Study the drawing (mm; zero at the part's minimum x, y, z) and answer. Round coordinates to 2 decimals unless told otherwise and drop trailing zeros. Order: outer loops, then holes, each group sorted by start corner. A loop starts at its lowest first (then second) coordinate and runs counter-clockwise, first axis right, second up. Notation, with made-up numbers: M 87,39 L 129,39 A21 ccw 129,47 Z; hole C 84.25,61.25 d7. An arc over 180 degrees is marked long. Put each result on its own line as item: value. Start each with the question number.
1. The part is cut by section C-C (y = 1.5). Give the vertices of the cut face in (x, z), then the cut area to 3 significant figures.
2. The mould has two halves that part along X. Classify the marked faces 1, 2 and 3: +X half, -X half, draft (parallel to the pull), parting line (faces both ways), or undercut.
3. Consider line 1 (Z direction, x = 21.5, y = 4); line 2 (X direction, y = 10.75, z = 27.5); line 3 (X direction, y = 4, z = 18). Determine where each line is inside the solid, lowest interval first.
4. The part is cut by section B-B (z = 13.5). Give the vertices of the cut face in (x, y), then the cut area to 3 significant figures.
5. Each of these flat-tipped pins is pushed along its axis until it touches: pin 1 Ø6 at (y, z) = (4, 35) entering from -X; pin 2 Ø2 at (x, y) = (37.5, 8.5) entering from +Z; pin 3 Ø2 at (y, z) = (11.5, 15.5) entering from -X; pin 4 Ø19 at (x, z) = (16, 23) entering from -Y. Where does it stop, or does it pass through?
6. The part is cut by section A-A (x = 15.5). Give the vertices of the cut face in (y, z).
7. The part is cut by section D-D (y = 12.25). Give the vertices of the cut face in (x, z), then the cut area to 3 significant figures.
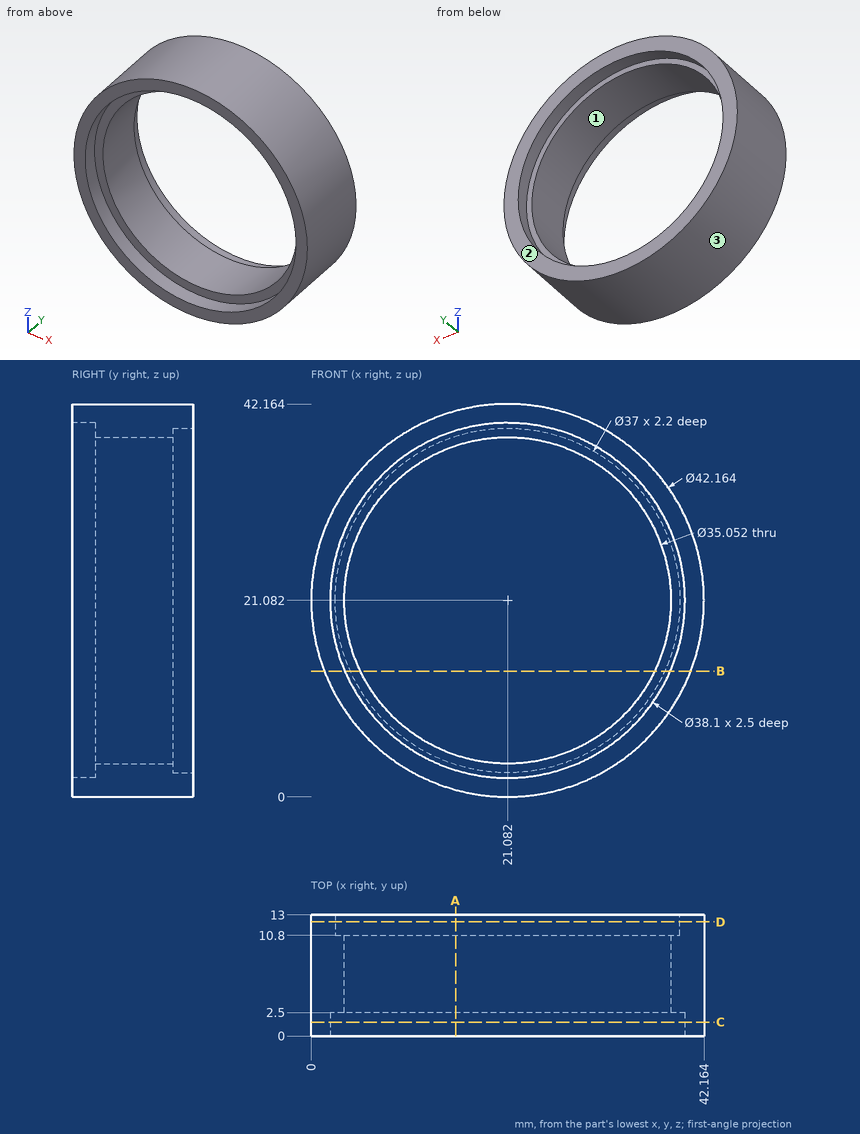
Resolved:
1. outline: C 21.08,21.08 d42.16; hole C 21.08,21.08 d38.1
1. area: 256 mm2
2. face 1: undercut
2. face 2: draft
2. face 3: parting line
3. line 1: 0 to 3.56, 38.6 to 42.16
3. line 2: 1 to 4.77, 37.39 to 41.16
3. line 3: 0.23 to 3.83, 38.33 to 41.94
4. outline: M 1.41,0 L 3.61,0 L 3.61,2.5 L 5.28,2.5 L 5.28,10.8 L 4.21,10.8 L 4.21,13 L 1.41,13 Z; M 36.88,2.5 L 38.56,2.5 L 38.56,0 L 40.75,0 L 40.75,13 L 37.96,13 L 37.96,10.8 L 36.88,10.8 Z
4. area: 87.5 mm2
5. pin 1: x = 3.05
5. pin 2: z = 35.46
5. pin 3: x = 0.5
5. pin 4: through
6. outline: M 0,0.75 L 13,0.75 L 13,3.44 L 10.8,3.44 L 10.8,4.47 L 2.5,4.47 L 2.5,2.87 L 0,2.87 Z; M 0,39.3 L 2.5,39.3 L 2.5,37.7 L 10.8,37.7 L 10.8,38.72 L 13,38.72 L 13,41.41 L 0,41.41 Z
7. outline: C 21.08,21.08 d42.16; hole C 21.08,21.08 d37
7. area: 321 mm2
